For this review, take the finished solid that the model builds, in its own axes (mm). A direction names the side the tool comes from. Give positions to 0.01 mm unless a question says otherwise; leave off trailing zeros. Write each loop counter-clockwise with the first axis right and the second up, starting at its lowest first coordinate (ties: lowest second). Pieces come first, ordered by that corner, then holes.
Q1. Machinability: for faces 5 (the flat face through (2, 28, -44)), 6 (the flat face through (2, 1, -39)), 7 (the flat face through (2, 26.1, -41)), which of the approach directions +Z, -Z, +X, -X, +Y, -Y give a long, thin tool a straight path to every point of the face, cutting with its end or side? Answer none if there is none.
Q2. We need section A-A (y = 13.5). Write out the cut boundary in (x, z), then the cut area to 3 significant figures.
Q3. Insertion check: P1, Ø5, axis at y = 18, z = -117, coming from the +X side; P2, Ø1.3, axis at x = 3.5, z = -2.5, coming from the -Y side; P3, Ø5, axis at x = 3.5, z = -2.5, coming from the -Y side; P4, Ø2, axis at x = 4, z = -2.5, coming from the -Y side. Each pin has a flat end and moves straight along its axis. Give the tip position at first contact, or say it passes through.
Q4. Mouldability with a two-part tool opening along X and no side actions: class faces 1 (the cylindrical face through (5.248, 27.57, -0.713)), 2 (the cylindrical face through (3.588, 0.69, -43.498)), 3 (the flat face through (2, 1, -5)), 4 (the cylindrical face through (4.852, 28.31, -3.974)) as released by +X, released by -X, zero draft, split by the parting line, or undercut.
Q5. We need section B-B (z = -68.5). Write out the cut boundary in (x, y), then the cut area to 3 significant figures.
Q6. For line 1 (X direction, y = 0.4, z = -41.5); line 2 (X direction, y = 2, z = -41.5); line 3 (X direction, y = 2, z = -90.5), list the stretches that pass through material, from the lowest coordinate up.
```python
from build123d import *

# Parameters (mm, degrees)
SKETCH1_W           = 5
SKETCH1_H           = 147
BOSS_EXTRUDE1_DEPTH = 29
SKETCH2_W           = 5
SKETCH2_H           = 2.9
BOSS_EXTRUDE2_DEPTH = 6
SKETCH3_R           = 1.05
CUT_EXTRUDE1_DEPTH  = 150.953326072
SKETCH4_R           = 2
CUT_EXTRUDE2_DEPTH  = 1.4
FILLET1_R           = 4
FILLET2_R           = 2.5


with BuildPart() as part:
    # Sketch1 → Boss-Extrude1 (new body)
    with BuildSketch(Plane(origin=(0, 0, 0), x_dir=(1, 0, 0), z_dir=(0, 1, 0))):
        with Locations((-2.5, 73.5)):
            Rectangle(SKETCH1_W, SKETCH1_H)
    extrude(amount=BOSS_EXTRUDE1_DEPTH)

    # Sketch2 → Boss-Extrude2 (add)
    with BuildSketch(Plane(origin=(0, 0, 0), x_dir=(0, 0, -1), z_dir=(1, 0, 0))):
        with Locations((2.5, 27.55)):
            Rectangle(SKETCH2_W, SKETCH2_H)
        with Locations((41.5, 27.55)):
            Rectangle(SKETCH2_W, SKETCH2_H)
        with Locations((41.5, 1.45)):
            Rectangle(SKETCH2_W, SKETCH2_H)
        with Locations((2.5, 1.45)):
            Rectangle(SKETCH2_W, SKETCH2_H)
    extrude(amount=BOSS_EXTRUDE2_DEPTH)

    # Sketch3 → Cut-Extrude1 (cut, through all)
    with BuildSketch(Plane(origin=(0, 29, 0), x_dir=(1, 0, 0), z_dir=(0, 1, 0))):
        with Locations(Location((3.5, 41.5, 0), (0, 0, 270))):
            Circle(SKETCH3_R)
        with Locations(Location((3.5, 2.5, 0), (0, 0, 270))):
            Circle(SKETCH3_R)
    extrude(amount=-CUT_EXTRUDE1_DEPTH, mode=Mode.SUBTRACT)

    # Sketch4 → Cut-Extrude2 (cut)
    with BuildSketch(Plane(origin=(0, 29, 0), x_dir=(1, 0, 0), z_dir=(0, 1, 0))):
        with Locations(Location((3.5, 41.5, 0), (0, 0, 270))):
            Circle(SKETCH4_R)
        with Locations(Location((3.5, 2.5, 0), (0, 0, 270))):
            Circle(SKETCH4_R)
    cut_extrude2 = extrude(amount=-CUT_EXTRUDE2_DEPTH, mode=Mode.SUBTRACT)

    # Mirror2: Cut-Extrude2 across plane
    add(cut_extrude2.mirror(Plane.ZX.offset(14.5)), mode=Mode.SUBTRACT)

    # Fillet1
    fillet1_edges = [part.edges().sort_by_distance(p)[0] for p in [
        (-2.5, 0, -147),
        (-5, 14.5, 0),
        (-2.5, 29, -147),
    ]]
    fillet(fillet1_edges, radius=FILLET1_R)

    # Fillet2
    fillet2_edges = [part.edges().sort_by_distance(p)[0] for p in [
        (6, 1.45, -5),
        (6, 1.45, 0),
        (6, 1.45, -44),
        (6, 1.45, -39),
        (6, 27.55, -44),
        (6, 27.55, -39),
        (6, 27.55, -5),
        (6, 27.55, 0),
    ]]
    fillet(fillet2_edges, radius=FILLET2_R - 0.0001)  # a hair under: the kernel refuses the full size


solid = part.part
```
Computed:
1. face 5: -Z, +X, +Y, -Y
1. face 6: +X, +Y, -Y
1. face 7: +Z, -Z, +X
2. outline: (-5, -147) - (0, -147) - (0, 0) - (-1, 0) arc R4 ccw to (-5, -4) - close
2. area: 732 mm2
3. P1: stops at x = 0
3. P2: passes through
3. P3: stops at y = 0
3. P4: stops at y = 1.4
4. face 1: released by +X
4. face 2: undercut
4. face 3: zero draft
4. face 4: undercut
5. outline: (-5, 0) - (0, 0) - (0, 29) - (-5, 29) - close
5. area: 145 mm2
6. line 1: x = -5 to 1.5, 5.5 to 6
6. line 2: x = -5 to 2.45, 4.55 to 6
6. line 3: x = -5 to 0
